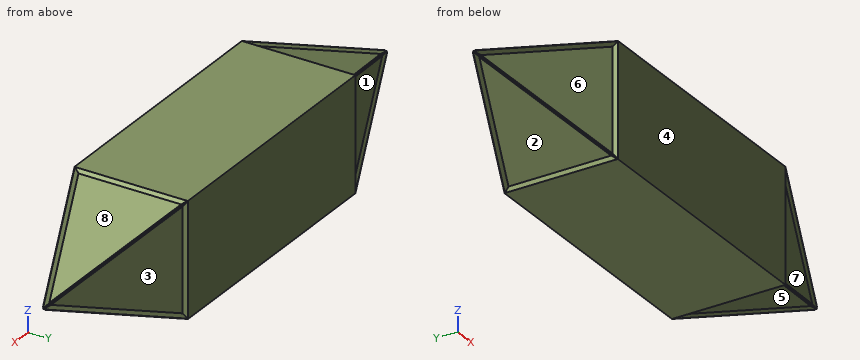
```python
from build123d import *

# Parameters (mm, degrees)
ESQUISSE3_W              = 1000
ESQUISSE3_H              = 430
BOSS_EXTRU_2_DEPTH       = 430
ESQUISSE4_W              = 430
ESQUISSE4_H              = 430
BOSS_EXTRU_3_DEPTH       = 522.4
BOSS_EXTRU_3_TAPER       = 22
ESQUISSE5_W              = 430
ESQUISSE5_H              = 430
BOSS_EXTRU_4_DEPTH       = 522
BOSS_EXTRU_4_TAPER       = 22
ENL_V_MAT_EXTRU_1_DEPTH  = 10
ENL_V_MAT_EXTRU_1_TAPER  = 53
ENL_V_MAT_EXTRU_2_DEPTH  = 10
ENL_V_MAT_EXTRU_2_TAPER  = 53
ENL_V_MAT_EXTRU_3_DEPTH  = 10
ENL_V_MAT_EXTRU_3_TAPER  = 53
ENL_V_MAT_EXTRU_4_DEPTH  = 10
ENL_V_MAT_EXTRU_4_TAPER  = 53
ENL_V_MAT_EXTRU_7_DEPTH  = 10
ENL_V_MAT_EXTRU_7_TAPER  = 53
ENL_V_MAT_EXTRU_8_DEPTH  = 10
ENL_V_MAT_EXTRU_8_TAPER  = 53
ENL_V_MAT_EXTRU_9_DEPTH  = 10
ENL_V_MAT_EXTRU_9_TAPER  = 53
ENL_V_MAT_EXTRU_10_DEPTH = 10
ENL_V_MAT_EXTRU_10_TAPER = 53


with BuildPart() as part:
    # Esquisse3 → Boss.-Extru.2 (new body)
    with BuildSketch(Plane.XY):
        with Locations((500, 215)):
            Rectangle(ESQUISSE3_W, ESQUISSE3_H)
    extrude(amount=BOSS_EXTRU_2_DEPTH)

    # Esquisse4 → Boss.-Extru.3 (add)
    with BuildSketch(Plane.ZY):
        with Locations((215, 215)):
            Rectangle(ESQUISSE4_W, ESQUISSE4_H)
    extrude(amount=BOSS_EXTRU_3_DEPTH, taper=BOSS_EXTRU_3_TAPER)

    # Esquisse5 → Boss.-Extru.4 (add)
    with BuildSketch(Plane(origin=(1000, 0, 0), x_dir=(0, 0, -1), z_dir=(1, 0, 0))):
        with Locations((-215, 215)):
            Rectangle(ESQUISSE5_W, ESQUISSE5_H)
    extrude(amount=BOSS_EXTRU_4_DEPTH, taper=BOSS_EXTRU_4_TAPER)

    # Esquisse6 → Enlèv. mat.-Extru.1 (cut)
    with BuildSketch(Plane(origin=(-149.351549649, 0, 369.658057073), x_dir=(0.927183855, 0, 0.374606593), z_dir=(-0.374606593, 0, 0.927183855))):
        Polygon((160.080835169, 428.557531009), (-410.003981176, 215), (160.080835169, 1.442468991), align=None)
    extrude(amount=-ENL_V_MAT_EXTRU_1_DEPTH, taper=ENL_V_MAT_EXTRU_1_TAPER, mode=Mode.SUBTRACT)

    # Esquisse7 → Enlèv. mat.-Extru.2 (cut)
    with BuildSketch(Plane(origin=(-149.351549649, 369.658057073, 0), x_dir=(0.927183855, 0.374606593, 0), z_dir=(-0.374606593, 0.927183855, 0))):
        Polygon((160.080835169, -428.557531009), (160.080835169, -1.442468991), (-410.003981176, -215), align=None)
    extrude(amount=-ENL_V_MAT_EXTRU_2_DEPTH, taper=ENL_V_MAT_EXTRU_2_TAPER, mode=Mode.SUBTRACT)

    # Esquisse8 → Enlèv. mat.-Extru.3 (cut)
    with BuildSketch(Plane(origin=(0, 0, 0), x_dir=(-0.927183855, 0, 0.374606593), z_dir=(-0.374606593, 0, -0.927183855))):
        Polygon((1, 428.557531009), (1, 1.442468991), (571.084816345, 215), align=None)
    extrude(amount=-ENL_V_MAT_EXTRU_3_DEPTH, taper=ENL_V_MAT_EXTRU_3_TAPER, mode=Mode.SUBTRACT)

    # Esquisse9 → Enlèv. mat.-Extru.4 (cut)
    with BuildSketch(Plane(origin=(0, 0, 0), x_dir=(0.927183855, -0.374606593, 0), z_dir=(-0.374606593, -0.927183855, 0))):
        Polygon((-571.084816345, 215), (-1, 1.442468991), (-1, 428.557531009), align=None)
    extrude(amount=-ENL_V_MAT_EXTRU_4_DEPTH, taper=ENL_V_MAT_EXTRU_4_TAPER, mode=Mode.SUBTRACT)

    # Esquisse12 → Enlèv. mat.-Extru.7 (cut)
    with BuildSketch(Plane(origin=(140.330099831, -347.329185229, 0), x_dir=(-0.927183855, -0.374606593, 0), z_dir=(0.374606593, -0.927183855, 0))):
        Polygon((-928.183854567, -428.557531009), (-928.183854567, -1.442468991), (-1498.268670912, -215), align=None)
    extrude(amount=-ENL_V_MAT_EXTRU_7_DEPTH, taper=ENL_V_MAT_EXTRU_7_TAPER, mode=Mode.SUBTRACT)

    # Esquisse13 → Enlèv. mat.-Extru.8 (cut)
    with BuildSketch(Plane(origin=(289.681649479, 0, 716.987242302), x_dir=(0.927183855, 0, -0.374606593), z_dir=(0.374606593, 0, 0.927183855))):
        Polygon((767.103019398, 428.557531009), (767.103019398, 1.442468991), (1337.187835743, 215), align=None)
    extrude(amount=-ENL_V_MAT_EXTRU_8_DEPTH, taper=ENL_V_MAT_EXTRU_8_TAPER, mode=Mode.SUBTRACT)

    # Esquisse14 → Enlèv. mat.-Extru.9 (cut)
    with BuildSketch(Plane(origin=(289.681649479, 716.987242302, 0), x_dir=(0.927183855, -0.374606593, 0), z_dir=(0.374606593, 0.927183855, 0))):
        Polygon((767.103019398, -1.442468991), (767.103019398, -428.557531009), (1337.187835743, -215), align=None)
    extrude(amount=-ENL_V_MAT_EXTRU_9_DEPTH, taper=ENL_V_MAT_EXTRU_9_TAPER, mode=Mode.SUBTRACT)

    # Esquisse15 → Enlèv. mat.-Extru.10 (cut)
    with BuildSketch(Plane(origin=(140.330099831, 0, -347.329185229), x_dir=(-0.927183855, 0, -0.374606593), z_dir=(0.374606593, 0, -0.927183855))):
        Polygon((-928.183854567, 428.557531009), (-1498.268670912, 215), (-928.183854567, 1.442468991), align=None)
    extrude(amount=-ENL_V_MAT_EXTRU_10_DEPTH, taper=ENL_V_MAT_EXTRU_10_TAPER, mode=Mode.SUBTRACT)


solid = part.part
```
Could you check a few things on this model? Use its own coordinates, in mm. Face numbers are marked on the shaded views. A direction names the side the tool comes from. Give positions to 0.01 mm unless a question says otherwise; leave off trailing zeros.
Q1. I'm going to push flat-ended pins straight in: P1, Ø1.5, axis at y = 134.5, z = 370, coming from the +X side; P2, Ø1.5, axis at x = 1094, z = 193.5, coming from the -Y side; P3, Ø12, axis at y = 277.5, z = 366.5, coming from the +X side. Where does each tip first touch, or does it pass through?
Q2. We'd pull the mould along Z, two halves only. Please class the marked faces 1, 2, 3 and 4: +Z half, -Z half, draft (parallel to the pull), parting line (faces both ways), or undercut.
Q3. If I drill on line 1 along X through (y, z) = (57.5, 338); line 2 along X through (y, z) = (290, 113); line 3 along Z through (x, y) = (-393.5, 240), over which ranges is the centre line in solid material (lowest first)?
Q4. For the marked faces 5, 6, 7 and 8, which set-ups out of +Z, -Z, +X, -X, +Y, -Y let a thin tool reach every point of the face, with its end or its side?
Solution:
1. P1: stops at x = 1123.67
1. P2: stops at y = 48.46
1. P3: stops at x = 1145.32
2. face 1: undercut
2. face 2: -Z half
2. face 3: undercut
2. face 4: draft
3. line 1: x = -115.62 to 1115.62
3. line 2: x = -252.99 to 1252.99
3. line 3: z = 169.77 to 260.23
4. face 5: -Z, +X
4. face 6: -X, -Y
4. face 7: +X, -Y
4. face 8: +Z, +X
